Work out the finished part from the listing and answer in its coordinate system (mm). A direction names the side the tool comes from. Coordinates: 2 decimals unless noted, no trailing zeros. Order: outer loops, then holes, each group sorted by start corner. A loop starts at its lowest first (then second) coordinate and runs counter-clockwise, first axis right, second up.
1. Flat-ended cylindrical pins translate along their axes: pin 1 Ø1 at (x, y) = (7, 16) entering from -Z; pin 2 Ø1.5 at (y, z) = (24.5, 4) entering from +X; pin 3 Ø3 at (y, z) = (23, 0.5) entering from -X. Find the tip coordinate at first contact, or state that the pin passes through.
2. The part is cut by section A-A, the plane x = 0. Give the vertices of the cut face in (y, z), then the cut area to 3 significant figures.
3. A tool of negligible diameter and unlimited length cuts with its end or side. For faces 1 (the flat face through (2.75, 22, -4)), 2 (the cylindrical face through (-5.158, 1.726, -3.955)), 3 (the flat face through (0, 22, 5.75)), 4 (the flat face through (0, 22, -5.75)), from which of +Z, -Z, +X, -X, +Y, -Y can it reach the whole face along a straight path? Write none if from no direction.
4. The part is cut by section B-B, the plane z = 0. Give the vertices of the cut face in (x, y), then the cut area to 3 significant figures.
5. The part is cut by section C-C, the plane y = 25.5. Give the vertices of the cut face in (x, z).
6. The part is cut by section D-D, the plane z = -11. Give the vertices of the cut face in (x, y).
7. Determine the mould class of faces 5 (the flat face through (-4, 22, -2.75)), 6 (the flat face through (3, 3.5, 0)), 7 (the flat face through (0, 3, 27)) for opening direction Z: +Z half, -Z half, draft (parallel to the pull), parting line (faces both ways), or undercut.
8. Find the intervals of material crossed by probe 1 along Z at (x, y) = (0, 11.25); probe 2 along Z at (x, y) = (0, 0.8); probe 3 along X at (y, z) = (21, 0), in increasing order.
```python
from build123d import *

# Parameters (mm, degrees)
SKETCH1_R           = 30
EXTRUDE_C_DEPTH     = 3
SKETCH2_R           = 26.5
BOSS_EXTRUDE2_DEPTH = 6
SKETCH3_R           = 30
BOSS_EXTRUDE3_DEPTH = 3
SKETCH4_W           = 5.5
SKETCH4_H           = 3
SKETCH4_W_2         = 3
SKETCH4_H_2         = 5.5
BOSS_EXTRUDE4_DEPTH = 16
SKETCH5_R           = 10
BOSS_EXTRUDE5_DEPTH = 4
SKETCH7_R           = 2.25
CUT_EXTRUDE1_DEPTH  = 46
SKETCH8_R           = 6.5
CUT_EXTRUDE2_DEPTH  = 3.5


with BuildPart() as part:
    # Sketch1 → Extrude c (new body)
    with BuildSketch(Plane(origin=(0, 0, 0), x_dir=(1, 0, 0), z_dir=(0, 1, 0))):
        Circle(SKETCH1_R)
    extrude(amount=EXTRUDE_C_DEPTH)

    # Sketch2 → Boss-Extrude2 (add)
    with BuildSketch(Plane(origin=(0, 3, 0), x_dir=(1, 0, 0), z_dir=(0, 1, 0))):
        Circle(SKETCH2_R)
    extrude(amount=BOSS_EXTRUDE2_DEPTH)

    # Sketch3 → Boss-Extrude3 (add)
    with BuildSketch(Plane(origin=(0, 9, 0), x_dir=(1, 0, 0), z_dir=(0, 1, 0))):
        Circle(SKETCH3_R)
    extrude(amount=BOSS_EXTRUDE3_DEPTH)

    # Sketch4 → Boss-Extrude4 (add)
    with BuildSketch(Plane(origin=(0, 12, 0), x_dir=(1, 0, 0), z_dir=(0, 1, 0))):
        with Locations((0, 4.25)):
            Rectangle(SKETCH4_W, SKETCH4_H)
        with Locations((-4.25, 0)):
            Rectangle(SKETCH4_W_2, SKETCH4_H_2)
        Rectangle(SKETCH4_W, SKETCH4_H_2)
        with Locations((0, -4.25)):
            Rectangle(SKETCH4_W, SKETCH4_H)
        with Locations((4.25, 0)):
            Rectangle(SKETCH4_W_2, SKETCH4_H_2)
    extrude(amount=BOSS_EXTRUDE4_DEPTH)

    # Sketch5 → Boss-Extrude5 (add)
    with BuildSketch(Plane(origin=(0, 12, 0), x_dir=(1, 0, 0), z_dir=(0, 1, 0))):
        Circle(SKETCH5_R)
    extrude(amount=BOSS_EXTRUDE5_DEPTH)

    # Sketch7 → Cut-Extrude1 (cut)
    with BuildSketch(Plane(origin=(0, 28, 0), x_dir=(1, 0, 0), z_dir=(0, 1, 0))):
        Circle(SKETCH7_R)
    extrude(amount=-CUT_EXTRUDE1_DEPTH, mode=Mode.SUBTRACT)

    # Sketch8 → Cut-Extrude2 (cut)
    with BuildSketch(Plane.XZ):
        Circle(SKETCH8_R)
    extrude(amount=-CUT_EXTRUDE2_DEPTH, mode=Mode.SUBTRACT)


solid = part.part
```
Geometry says:
1. pin 1: stops at z = -7.6
1. pin 2: stops at x = 2.75
1. pin 3: stops at x = -5.75
2. outline: (0, -30) - (3, -30) - (3, -26.5) - (9, -26.5) - (9, -30) - (12, -30) - (12, -10) - (16, -10) - (16, -5.75) - (28, -5.75) - (28, -2.25) - (3.5, -2.25) - (3.5, -6.5) - (0, -6.5) - close; (0, 6.5) - (3.5, 6.5) - (3.5, 2.25) - (28, 2.25) - (28, 5.75) - (16, 5.75) - (16, 10) - (12, 10) - (12, 30) - (9, 30) - (9, 26.5) - (3, 26.5) - (3, 30) - (0, 30) - close
2. area: 740 mm2
3. face 1: -Z, +X, +Y
3. face 2: -Y
3. face 3: +Z, +X, -X, +Y
3. face 4: -Z, +X, -X, +Y
4. outline: (-30, 0) - (-6.5, 0) - (-6.5, 3.5) - (-2.25, 3.5) - (-2.25, 28) - (-5.75, 28) - (-5.75, 16) - (-10, 16) - (-10, 12) - (-30, 12) - (-30, 9) - (-26.5, 9) - (-26.5, 3) - (-30, 3) - close; (2.25, 3.5) - (6.5, 3.5) - (6.5, 0) - (30, 0) - (30, 3) - (26.5, 3) - (26.5, 9) - (30, 9) - (30, 12) - (10, 12) - (10, 16) - (5.75, 16) - (5.75, 28) - (2.25, 28) - close
4. area: 740 mm2
5. outline: (-5.75, -2.75) - (-2.75, -2.75) - (-2.75, -5.75) - (2.75, -5.75) - (2.75, -2.75) - (5.75, -2.75) - (5.75, 2.75) - (2.75, 2.75) - (2.75, 5.75) - (-2.75, 5.75) - (-2.75, 2.75) - (-5.75, 2.75) - close; hole circle Ø4.5 at (0, 0)
6. outline: (-27.91, 0) - (27.91, 0) - (27.91, 3) - (24.11, 3) - (24.11, 9) - (27.91, 9) - (27.91, 12) - (-27.91, 12) - (-27.91, 9) - (-24.11, 9) - (-24.11, 3) - (-27.91, 3) - close
7. face 5: -Z half
7. face 6: undercut
7. face 7: draft
8. probe 1: z = -30 to -2.25, 2.25 to 30
8. probe 2: z = -30 to -6.5, 6.5 to 30
8. probe 3: x = -5.75 to -2.25, 2.25 to 5.75
